from build123d import *

# Parameters (mm, degrees)
ESQUISSE1_R                  = 12.5
BOSS_EXTRU_1_DEPTH           = 16
ESQUISSE2_R                  = 1
BOSS_EXTRU_2_DEPTH           = 8
BOSS_EXTRU_3_DEPTH           = 4
ESQUISSE5_R                  = 1.5
ENL_V_MAT_EXTRU_1_DEPTH      = 5
R_P_TITION_CIRCULAIRE1_COUNT = 3
ESQUISSE6_R                  = 6
BOSS_EXTRU_4_DEPTH           = 1


with BuildPart() as part:
    # Esquisse1 → Boss.-Extru.1 (new body)
    with BuildSketch(Plane(origin=(0, 0, 0), x_dir=(1, 0, 0), z_dir=(0, 1, 0))):
        with Locations(Location((0, 0, 0), (0, 0, 270))):
            Circle(ESQUISSE1_R)
    extrude(amount=BOSS_EXTRU_1_DEPTH)

    # Esquisse2 → Boss.-Extru.2 (add)
    with BuildSketch(Plane(origin=(0, 16, 0), x_dir=(1, 0, 0), z_dir=(0, 1, 0))):
        with Locations(Location((0, 0, 0), (0, 0, 270))):
            Circle(ESQUISSE2_R)
    extrude(amount=BOSS_EXTRU_2_DEPTH)

    # Esquisse4 → Boss.-Extru.3 (add)
    with BuildSketch(Plane.XZ):
        Polygon((0, 20.790629037), (2, 20.790629037), (2, 9.492710375), (0, 9.492710375), (-2, 9.492710375), (-2, 20.790629037), align=None)
    extrude(amount=-BOSS_EXTRU_3_DEPTH)

    # Esquisse5 → Enlèv. mat.-Extru.1 (cut)
    with BuildSketch(Plane(origin=(0, 16, 0), x_dir=(1, 0, 0), z_dir=(0, 1, 0))):
        with Locations(Location((0, 9, 0), (0, 0, 270))):
            Circle(ESQUISSE5_R)
    enl_v_mat_extru_1 = extrude(amount=-ENL_V_MAT_EXTRU_1_DEPTH, mode=Mode.SUBTRACT)

    # Répétition circulaire1: Enlèv. mat.-Extru.1 ×3 about axis
    r_p_tition_circulaire1_axis = Axis((0, 0, 0), (0, 1, 0))
    for i in range(1, R_P_TITION_CIRCULAIRE1_COUNT):
        add(enl_v_mat_extru_1.rotate(r_p_tition_circulaire1_axis, i * 360 / R_P_TITION_CIRCULAIRE1_COUNT), mode=Mode.SUBTRACT)

    # Esquisse6 → Boss.-Extru.4 (add)
    with BuildSketch(Plane(origin=(0, 16, 0), x_dir=(1, 0, 0), z_dir=(0, 1, 0))):
        with Locations(Location((0, 0, 0), (0, 0, 270))):
            Circle(ESQUISSE6_R)
    extrude(amount=BOSS_EXTRU_4_DEPTH)


solid = part.part
The model under review builds one solid part; all positions refer to its coordinate system, in mm. A direction names the side the tool comes from. Coordinates: 2 decimals unless noted, no trailing zeros. Loops run counter-clockwise (first coordinate to the right, second up) from the corner with the lowest first, then second, coordinate; pieces in that order, holes last.
(1) Tool access review of faces 1 (the flat face through (0, 24, 0)), 2 (the flat face through (2, 2, 17)), 3 (the flat face through (8, 11, 5)): name each direction out of +Z, -Z, +X, -X, +Y, -Y from which nothing blocks a thin tool from reaching the whole face with its end or side.
Determined:
face 1: +Z, -Z, +X, -X, +Y
face 2: +Z, +X, +Y, -Y
face 3: +Y
(2) Draft analysis for pull direction Z (two halves, no side actions). For faces 4 (the cylindrical face through (3.755, 7.888, 11.923)), 5 (the flat face through (-2, 2, 17)), 6 (the cylindrical face through (0.07, 13.54, -10.5)), state which applies: +Z half, -Z half, draft (parallel to the pull), parting line (faces both ways), or undercut.
Determined:
face 4: parting line
face 5: draft
face 6: undercut
(3) Insertion check: P1, Ø8, axis at x = 6.5, z = -6.5, coming from the +Y side; P2, Ø8, axis at y = 6.5, z = 17.5, coming from the -X side; P3, Ø0.9, axis at x = -8, z = 4, coming from the +Y side. Each pin has a flat end and moves straight along its axis. Give the tip position at first contact, or say it passes through.
Determined:
P1: stops at y = 17
P2: stops at x = -2
P3: stops at y = 11
(4) Wall thickness on L1, parallel to X at y = 14.9, z = 4.5; L2, parallel to Y at x = 8, z = 6.5; L3, parallel to Y at x = 1.5, z = -0.5: over which ranges is each line inside the solid? List them lowest first.
Determined:
L1: x = -11.66 to -9.29, -6.29 to 6.29, 9.29 to 11.66
L2: y = 0 to 16
L3: y = 0 to 17
(5) Consider section A-A, the plane z = 0. Give the boundary of the cut face in (x, y), plus the area to 3 significant figures.
Determined:
outline: (-12.5, 0) - (12.5, 0) - (12.5, 16) - (6, 16) - (6, 17) - (1, 17) - (1, 24) - (-1, 24) - (-1, 17) - (-6, 17) - (-6, 16) - (-12.5, 16) - close
area: 426 mm2
(6) Consider section D-D, the plane z = -10. Give the boundary of the cut face in (x, y).
Determined:
outline: (-7.5, 0) - (7.5, 0) - (7.5, 16) - (1.12, 16) - (1.12, 11) - (-1.12, 11) - (-1.12, 16) - (-7.5, 16) - close
(7) Consider section C-C, the plane y = 21.5. Give the boundary of the cut face in (x, z).
Determined:
outline: circle Ø2 at (0, 0)
(8) Consider section B-B, the plane x = -8.75. Give the boundary of the cut face in (y, z), plus the area to 3 significant figures.
Determined:
outline: (0, -8.93) - (16, -8.93) - (16, 3.34) - (11, 3.34) - (11, 5.66) - (16, 5.66) - (16, 8.93) - (0, 8.93) - close
area: 274 mm2
